The model under review builds one solid part; all positions refer to its coordinate system, in mm. A direction names the side the tool comes from. Round coordinates to 2 decimals unless told otherwise and drop trailing zeros. Order: outer loops, then holes, each group sorted by start corner. A loop starts at its lowest first (then second) coordinate and runs counter-clockwise, first axis right, second up. Notation, with made-up numbers: (17.25, 12.25) - (50.25, 12.25) arc R14 ccw to (50.25, 18.25) - close; hole circle Ø1 at (-0.5, -13). An arc over 180 degrees is marked (long way). One line per question, with ' | ' between items. Start each with the question number.
Item 1: For L1, parallel to X at y = 15.5, z = -2; L2, parallel to X at y = 8, z = 8.5; L3, parallel to Y at x = 42, z = -6.5, list the stretches that pass through material, from the lowest coordinate up. Write a range as [from, to].
Item 2: Draft analysis for pull direction X (two halves, no side actions). For faces 6 (the face through (41, -12, -6)), 7 (the face through (-36.651, -15, -7)), 8 (the face through (50, -27, 1)), state which applies: +X half, -X half, draft (parallel to the pull), parting line (faces both ways), or undercut.
Item 3: Insertion check: pin 1 Ø3 at (x, y) = (-14, 33) entering from -Z; pin 2 Ø4 at (x, z) = (43.5, -9.5) entering from +Y; pin 3 Ø2 at (x, y) = (32, -14) entering from -Z. Each pin has a flat end and moves straight along its axis. Give the tip position at first contact, or say it passes through.
Item 4: Add section B-B on y = 13.5. State the section outline as (x, z) points, and give its area (3 significant figures).
Item 5: Add section C-C on z = -16.5. State the section outline as (x, y) points, and give its area (3 significant figures).
Item 6: Tool access review of faces 1 (the face through (0, -83, -20.598)), 2 (the face through (0, 27.5, 2)), 3 (the face through (-38, -14, -1)), 4 (the face through (-45, 15, -13)), 5 (the face through (-1, -48, 0)): name each direction out of +Z, -Z, +X, -X, +Y, -Y from which nothing blocks a thin tool from reaching the whole face with its end or side.
Item 7: Add section D-D on y = -40.5. State the section outline as (x, z) points, and give its area (3 significant figures).
Item 8: Add section A-A on x = -28.5. State the section outline as (y, z) points, and give its area (3 significant figures).
from build123d import *

# Parameters (mm, degrees)
SKETCH_1_W          = 100
SKETCH_1_H          = 100
EXTRUDE_1_DEPTH     = 10
SKETCH_2_W          = 65
SKETCH_2_H          = 55
CUT_EXTRUDE_1_DEPTH = 11
SKETCH_3_W          = 88
SKETCH_3_H          = 88
CUT_EXTRUDE_2_DEPTH = 7
SKETCH_4_W          = 100
SKETCH_4_H          = 38
EXTRUDE_2_DEPTH     = 35
SKETCH_8_W          = 100
SKETCH_8_H          = 25
CUT_EXTRUDE_3_DEPTH = 30
SKETCH_9_W          = 17.5
SKETCH_9_H          = 5
EXTRUDE_3_DEPTH     = 13
SKETCH_10_W         = 2.733389199
SKETCH_10_H         = 5
CUT_EXTRUDE_5_DEPTH = 12
SKETCH_11_W         = 32.468839848
SKETCH_11_H         = 16.671988928
CUT_EXTRUDE_6_DEPTH = 12


with BuildPart() as part:
    # 草图1 → 凸台-拉伸1 (new body)
    with BuildSketch(Plane.XY):
        Rectangle(SKETCH_1_W, SKETCH_1_H)
    extrude(amount=EXTRUDE_1_DEPTH)

    # 草图2 → 切除-拉伸1 (cut, through all)
    with BuildSketch(Plane.XY.offset(10)):
        Rectangle(SKETCH_2_W, SKETCH_2_H)
    extrude(amount=-CUT_EXTRUDE_1_DEPTH, mode=Mode.SUBTRACT)

    # 草图3 → 切除-拉伸2 (cut)
    with BuildSketch(Plane.XY.offset(10)):
        Rectangle(SKETCH_3_W, SKETCH_3_H)
    extrude(amount=-CUT_EXTRUDE_2_DEPTH, mode=Mode.SUBTRACT)

    # 草图4 → 凸台-拉伸2 (add)
    with BuildSketch(Plane.XZ.offset(50)):
        with Locations((0, -9)):
            Rectangle(SKETCH_4_W, SKETCH_4_H)
    extrude(amount=EXTRUDE_2_DEPTH)

    # 草图8 → 切除-拉伸3 (cut)
    with BuildSketch(Plane(origin=(0, -50, 0), x_dir=(1, 0, 0), z_dir=(0, 1, 0))):
        with Locations((0, 12.5)):
            Rectangle(SKETCH_8_W, SKETCH_8_H)
    extrude(amount=-CUT_EXTRUDE_3_DEPTH, mode=Mode.SUBTRACT)

    # 草图9 → 凸台-拉伸3 (add)
    with BuildSketch(Plane(origin=(0, 0, 0), x_dir=(-1, 0, 0), z_dir=(0, 0, -1))):
        with Locations((-41.25, 14.5)):
            Rectangle(SKETCH_9_W, SKETCH_9_H)
        with Locations((-41.25, -14.5)):
            Rectangle(SKETCH_9_W, SKETCH_9_H)
        with Locations((41.25, 14.5)):
            Rectangle(SKETCH_9_W, SKETCH_9_H)
        with Locations((41.25, -14.5)):
            Rectangle(SKETCH_9_W, SKETCH_9_H)
    extrude(amount=EXTRUDE_3_DEPTH)

    # 草图10 → 切除-拉伸5 (cut)
    with BuildSketch(Plane(origin=(0, 0, -13), x_dir=(-1, 0, 0), z_dir=(0, 0, -1))):
        with Locations((-38.018129079, 14.5)):
            Rectangle(SKETCH_10_W, SKETCH_10_H)
        with Locations((-38.018129079, -14.5)):
            Rectangle(SKETCH_10_W, SKETCH_10_H)
        with Locations((38.018129079, -14.5)):
            Rectangle(SKETCH_10_W, SKETCH_10_H)
        with Locations((38.018129079, 14.5)):
            Rectangle(SKETCH_10_W, SKETCH_10_H)
    extrude(amount=-CUT_EXTRUDE_5_DEPTH, mode=Mode.SUBTRACT)

    # 草图11 → 切除-拉伸6 (cut)
    with BuildSketch(Plane.XZ.offset(85)):
        with Locations((0, -12.262013559)):
            Rectangle(SKETCH_11_W, SKETCH_11_H)
    extrude(amount=-CUT_EXTRUDE_6_DEPTH, mode=Mode.SUBTRACT)


solid = part.part
Determined:
1) L1: [-50, -39.38], [-36.65, -32.5], [32.5, 36.65], [39.38, 50] | L2: [-50, -44], [44, 50] | L3: [-85, -80], [-17, -12], [12, 17]
2) face 6: draft | face 7: undercut | face 8: +X half
3) pin 1: z = 0 | pin 2: y = 17 | pin 3: z = -13
4) outline: (-50, -13) - (-39.38, -13) - (-39.38, -1) - (-36.65, -1) - (-36.65, -13) - (-32.5, -13) - (-32.5, 3) - (-44, 3) - (-44, 10) - (-50, 10) - close; (32.5, -13) - (36.65, -13) - (36.65, -1) - (39.38, -1) - (39.38, -13) - (50, -13) - (50, 10) - (44, 10) - (44, 3) - (32.5, 3) - close | area: 578 mm2
5) outline: (-50, -85) - (-16.23, -85) - (-16.23, -80) - (-50, -80) - close; (16.23, -85) - (50, -85) - (50, -80) - (16.23, -80) - close | area: 338 mm2
6) face 1: +Y, -Y | face 2: +Z, -Z | face 3: -Z, +Y | face 4: -Z, +X, -X, +Y | face 5: +X, -X
7) outline: (-50, 0) - (50, 0) - (50, 10) - (44, 10) - (44, 3) - (-44, 3) - (-44, 10) - (-50, 10) - close | area: 384 mm2
8) outline: (-85, -28) - (-50, -28) - (-50, -25) - (-80, -25) - (-80, 0) - (-27.5, 0) - (-27.5, 3) - (-44, 3) - (-44, 10) - (-85, 10) - close; (27.5, 0) - (50, 0) - (50, 10) - (44, 10) - (44, 3) - (27.5, 3) - close | area: 799 mm2
